from build123d import *

# Parameters (mm, degrees)
SKETCH_1_W                  = 125
SKETCH_1_H                  = 20
EXTRUDE_1_DEPTH             = 10
CUT_EXTRUDE_1_DEPTH         = 3.5
CUT_EXTRUDE_2_DEPTH         = 3.5
CUT_EXTRUDE_3_DEPTH         = 3.5
CUT_EXTRUDE_4_DEPTH         = 3.5
CUT_EXTRUDE_5_DEPTH         = 3.5
CUT_EXTRUDE_6_DEPTH         = 3.5
HOLE_WIZARD_8_7_8_7_1_D     = 8.7
HOLE_WIZARD_8_7_8_7_1_DEPTH = 10
HOLE_WIZARD_8_5_8_5_1_D     = 8.5
HOLE_WIZARD_8_5_8_5_1_DEPTH = 10
HOLE_WIZARD_8_3_8_3_1_D     = 8.3
HOLE_WIZARD_8_3_8_3_1_DEPTH = 10
FILLET_1_R                  = 5


with BuildPart() as part:
    # 草图1 → 凸台-拉伸1 (new body)
    with BuildSketch(Plane(origin=(0, 0, 0), x_dir=(-1, 0, 0), z_dir=(0, 0, -1))):
        with Locations((-62.5, -116)):
            Rectangle(SKETCH_1_W, SKETCH_1_H)
    extrude(amount=-EXTRUDE_1_DEPTH)

    # 草图2 → 切除-拉伸1 (cut)
    with BuildSketch(Plane.XY.offset(10)):
        Polygon((93.85, -122.668395609), (97.7, -116), (93.85, -109.331604391), (86.15, -109.331604391), (82.3, -116), (86.15, -122.668395609), align=None)
    extrude(amount=-CUT_EXTRUDE_1_DEPTH, mode=Mode.SUBTRACT)

    # 草图3 → 切除-拉伸2 (cut)
    with BuildSketch(Plane.XY.offset(10)):
        Polygon((73.825, -122.625094339), (77.65, -116), (73.825, -109.374905661), (66.175, -109.374905661), (62.35, -116), (66.175, -122.625094339), align=None)
    extrude(amount=-CUT_EXTRUDE_2_DEPTH, mode=Mode.SUBTRACT)

    # 草图4 → 切除-拉伸3 (cut)
    with BuildSketch(Plane.XY.offset(10)):
        Polygon((53.8, -122.581793069), (57.6, -116), (53.8, -109.418206931), (46.2, -109.418206931), (42.4, -116), (46.2, -122.581793069), align=None)
    extrude(amount=-CUT_EXTRUDE_3_DEPTH, mode=Mode.SUBTRACT)

    # 草图5 → 切除-拉伸4 (cut)
    with BuildSketch(Plane.XY.offset(10)):
        Polygon((33.775, -122.538491799), (37.55, -116), (33.775, -109.461508201), (26.225, -109.461508201), (22.45, -116), (26.225, -122.538491799), align=None)
    extrude(amount=-CUT_EXTRUDE_4_DEPTH, mode=Mode.SUBTRACT)

    # 草图6 → 切除-拉伸5 (cut)
    with BuildSketch(Plane.XY.offset(10)):
        Polygon((13.75, -122.495190528), (17.5, -116), (13.75, -109.504809472), (6.25, -109.504809472), (2.5, -116), (6.25, -122.495190528), align=None)
    extrude(amount=-CUT_EXTRUDE_5_DEPTH, mode=Mode.SUBTRACT)

    # 草图7 → 切除-拉伸6 (cut)
    with BuildSketch(Plane.XY.offset(10)):
        Polygon((113.875, -122.711696879), (117.75, -116), (113.875, -109.288303121), (106.125, -109.288303121), (102.25, -116), (106.125, -122.711696879), align=None)
    extrude(amount=-CUT_EXTRUDE_6_DEPTH, mode=Mode.SUBTRACT)

    # Ø8.7 (8.7) 直径孔1
    with Locations(Plane(origin=(0, 0, 0), x_dir=(-1, 0, 0), z_dir=(0, 0, -1))):
        with Locations((-110, -116)):
            Hole(HOLE_WIZARD_8_7_8_7_1_D / 2, depth=HOLE_WIZARD_8_7_8_7_1_DEPTH)

    # Ø8.5 (8.5) 直径孔1
    with Locations(Plane(origin=(0, 0, 0), x_dir=(-1, 0, 0), z_dir=(0, 0, -1))):
        with Locations((-70, -116), (-90, -116)):
            Hole(HOLE_WIZARD_8_5_8_5_1_D / 2, depth=HOLE_WIZARD_8_5_8_5_1_DEPTH)

    # Ø8.3 (8.3) 直径孔1
    with Locations(Plane(origin=(0, 0, 0), x_dir=(-1, 0, 0), z_dir=(0, 0, -1))):
        with Locations((-30, -116), (-50, -116), (-10, -116)):
            Hole(HOLE_WIZARD_8_3_8_3_1_D / 2, depth=HOLE_WIZARD_8_3_8_3_1_DEPTH)

    # 圆角1
    fillet_1_edges = [part.edges().sort_by_distance(p)[0] for p in [
        (125, -126, 5),
        (125, -106, 5),
    ]]
    fillet(fillet_1_edges, radius=FILLET_1_R)


solid = part.part
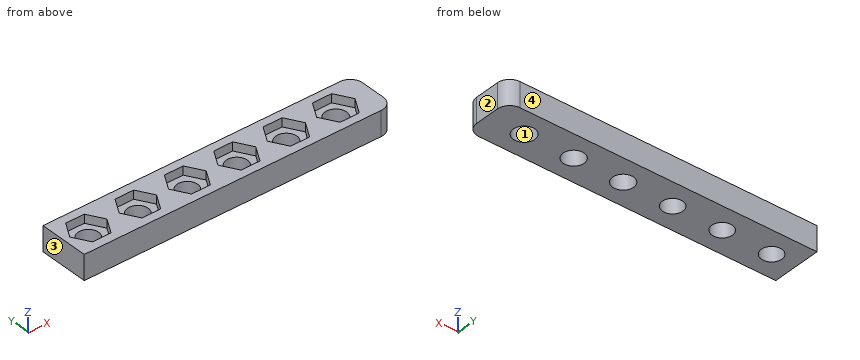
Could you check a few things on this model? Use its own coordinates, in mm. Face numbers are marked on the shaded views. Coordinates: 2 decimals unless noted, no trailing zeros. Order: outer loops, then holes, each group sorted by start corner. A loop starts at its lowest first (then second) coordinate and runs counter-clockwise, first axis right, second up. Notation, with made-up numbers: (-30, -7) -> (8, -7) arc R33 cw to (8, 25) -> close; hole circle Ø6 at (42.25, 40). An arc over 180 degrees is marked (long way). One line per item, written item: value. Start each with the question number.
1) Imagine slicing it at C-C on x = 30. List the corners of the cut face in (y, z) for me.
2) Imagine slicing it at B-B on z = 2. List the corners of the cut face in (x, y) for me, plus the area to 3 significant figures.
3) I'm going to push flat-ended pins straight in: pin 1 (4 mm diameter, centred on x = 28, y = -115, fed in from +Z); pin 2 (7 mm diameter, centred on x = 110, y = -116, fed in from +Z). Where does each tip first touch, or does it pass through?
4) Imagine slicing it at A-A on x = 70. List the corners of the cut face in (y, z) for me.
5) If I drill on L1, parallel to Y at x = 66.5, z = 6.75; L2, parallel to Y at x = 70, z = 5.25; L3, parallel to X at y = -121.5, z = 3.5, over which ranges is the centre line in solid material (lowest first)? Write a range as [from, to].
6) We'd pull the mould along X, two halves only. Please class the marked faces 1, 2, 3 and 4: +X half, -X half, draft (parallel to the pull), parting line (faces both ways), or undercut.
Answer list:
1. outline: (-126, 0) -> (-120.15, 0) -> (-120.15, 6.5) -> (-122.54, 6.5) -> (-122.54, 10) -> (-126, 10) -> close; (-111.85, 0) -> (-106, 0) -> (-106, 10) -> (-109.46, 10) -> (-109.46, 6.5) -> (-111.85, 6.5) -> close
2. outline: (0, -126) -> (120, -126) arc R5 ccw to (125, -121) -> (125, -111) arc R5 ccw to (120, -106) -> (0, -106) -> close; hole circle Ø8.3 at (10, -116); hole circle Ø8.3 at (30, -116); hole circle Ø8.3 at (50, -116); hole circle Ø8.5 at (70, -116); hole circle Ø8.5 at (90, -116); hole circle Ø8.7 at (110, -116)
2. area: 2,150 mm2
3. pin 1: stops at z = 6.5
3. pin 2: passes through
4. outline: (-126, 0) -> (-120.25, 0) -> (-120.25, 6.5) -> (-122.63, 6.5) -> (-122.63, 10) -> (-126, 10) -> close; (-111.75, 0) -> (-106, 0) -> (-106, 10) -> (-109.37, 10) -> (-109.37, 6.5) -> (-111.75, 6.5) -> close
5. L1: y = [-126, -122.63], [-109.37, -106]
5. L2: y = [-126, -120.25], [-111.75, -106]
5. L3: x = [0, 124.97]
6. face 1: undercut
6. face 2: +X half
6. face 3: -X half
6. face 4: draft
